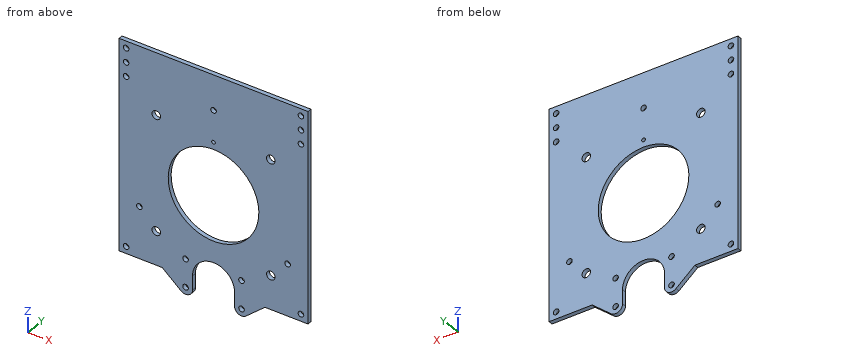
from build123d import *

# Parameters (mm, degrees)
SKETCH_1_R      = 2
SKETCH_1_R_2    = 3.05
SKETCH_1_R_3    = 1.3
SKETCH_1_R_4    = 32.4
EXTRUDE_1_DEPTH = 3


with BuildPart() as part:
    # ｽｹｯﾁ1 → ﾎﾞｽ - 押し出し1 (new body)
    with BuildSketch(Plane(origin=(0, 0, 0), x_dir=(1, 0, 0), z_dir=(0, 1, 0))):
        with BuildLine():
            Line((0, 150), (0, 0))
            Line((0, 0), (135, 0))
            Line((135, 0), (135, 150))
            Line((135, 150), (104.216771079, 150))
            Line((104.216771079, 150), (90.713938048, 161.330222216))
            ThreePointArc((90.713938048, 161.330222216), (85.386908691, 162.031538935), (82.5, 157.5))
            Line((82.5, 157.5), (82.5, 147.5))
            ThreePointArc((82.5, 147.5), (67.5, 132.5), (52.5, 147.5))
            Line((52.5, 147.5), (52.5, 150))
            Line((52.5, 150), (52.5, 157.5))
            ThreePointArc((52.5, 157.5), (49.613091309, 162.031538935), (44.286061952, 161.330222216))
            Line((44.286061952, 161.330222216), (30.783228921, 150))
            Line((30.783228921, 150), (0, 150))
        make_face()
        with Locations(Location((5, 5, 0), (0, 0, 270))):
            Circle(SKETCH_1_R, mode=Mode.SUBTRACT)
        with Locations(Location((5, 15, 0), (0, 0, 270))):
            Circle(SKETCH_1_R, mode=Mode.SUBTRACT)
        with Locations(Location((5, 25, 0), (0, 0, 270))):
            Circle(SKETCH_1_R, mode=Mode.SUBTRACT)
        with Locations(Location((26.558517369, 44.058517369, 0), (0, 0, 270))):
            Circle(SKETCH_1_R_2, mode=Mode.SUBTRACT)
        with Locations(Location((67.5, 25, 0), (0, 0, 270))):
            Circle(SKETCH_1_R, mode=Mode.SUBTRACT)
        with Locations(Location((130, 5, 0), (0, 0, 270))):
            Circle(SKETCH_1_R, mode=Mode.SUBTRACT)
        with Locations(Location((130, 15, 0), (0, 0, 270))):
            Circle(SKETCH_1_R, mode=Mode.SUBTRACT)
        with Locations(Location((130, 25, 0), (0, 0, 270))):
            Circle(SKETCH_1_R, mode=Mode.SUBTRACT)
        with Locations(Location((67.5, 47.5, 0), (0, 0, 270))):
            Circle(SKETCH_1_R_3, mode=Mode.SUBTRACT)
        with Locations(Location((108.441482631, 44.058517369, 0), (0, 0, 270))):
            Circle(SKETCH_1_R_2, mode=Mode.SUBTRACT)
        with Locations(Location((14.523144428, 113.168293767, 0), (0, 0, 270))):
            Circle(SKETCH_1_R, mode=Mode.SUBTRACT)
        with Locations(Location((67.5, 85, 0), (0, 0, 270))):
            Circle(SKETCH_1_R_4, mode=Mode.SUBTRACT)
        with Locations(Location((26.558517369, 125.941482631, 0), (0, 0, 270))):
            Circle(SKETCH_1_R_2, mode=Mode.SUBTRACT)
        with Locations(Location((5, 145, 0), (0, 0, 270))):
            Circle(SKETCH_1_R, mode=Mode.SUBTRACT)
        with Locations(Location((47.5, 137.5, 0), (0, 0, 270))):
            Circle(SKETCH_1_R, mode=Mode.SUBTRACT)
        with Locations(Location((47.5, 157.5, 0), (0, 0, 270))):
            Circle(SKETCH_1_R, mode=Mode.SUBTRACT)
        with Locations(Location((120.476855572, 113.168293767, 0), (0, 0, 270))):
            Circle(SKETCH_1_R, mode=Mode.SUBTRACT)
        with Locations(Location((87.5, 137.5, 0), (0, 0, 270))):
            Circle(SKETCH_1_R, mode=Mode.SUBTRACT)
        with Locations(Location((108.441482631, 125.941482631, 0), (0, 0, 270))):
            Circle(SKETCH_1_R_2, mode=Mode.SUBTRACT)
        with Locations(Location((130, 145, 0), (0, 0, 270))):
            Circle(SKETCH_1_R, mode=Mode.SUBTRACT)
        with Locations(Location((87.5, 157.5, 0), (0, 0, 270))):
            Circle(SKETCH_1_R, mode=Mode.SUBTRACT)
    extrude(amount=EXTRUDE_1_DEPTH)


solid = part.part
Work out the finished part from the listing and answer in its coordinate system (mm). Give positions to 0.01 mm unless a question says otherwise; leave off trailing zeros. Order: outer loops, then holes, each group sorted by start corner. A loop starts at its lowest first (then second) coordinate and runs counter-clockwise, first axis right, second up. Notation, with made-up numbers: (22.25, 13.25) -> (53.25, 13.25) arc R21 cw to (53.25, 45.25) -> close; hole circle Ø10 at (-30, 22.25). An arc over 180 degrees is marked (long way). Answer as a JSON object with one key per item and string values. Group by question number.
1. Consider line 1 along X through (y, z) = (2.15, -5); line 2 along X through (y, z) = (2.3, -125); line 3 along X through (y, z) = (2.4, -157.5). Determine where each line is inside the solid, lowest interval first. Write a range as [from, to].
2. Section B-B on x = 87.5 is taken. Determine the outline of the cut face in (y, z), plus the area to 3 significant figures.
3. Section D-D on z = -99.5 is taken. Determine the outline of the cut face in (x, y).
4. Section C-C on y = 0.75 is taken. Count the separate pieces of the cut face and the enclosed holes in it, plus the area to 3 significant figures.
5. Flat-ended cylindrical pins translate along their axes: pin 1 Ø3.5 at (x, z) = (26.56, -44.06) entering from +Y; pin 2 Ø0.9 at (y, z) = (1, -152.5) entering from +X; pin 3 Ø0.9 at (x, y) = (9.5, 1) entering from -Z. Find the tip coordinate at first contact, or state that the pin passes through.
6. Section A-A on z = -71 is taken. Determine the outline of the cut face in (x, y), plus the area to 3 significant figures.
Result sheet:
{
 "1": {"line 1": "x = [0, 3], [7, 128], [132, 135]", "line 2": "x = [0, 23.66], [29.46, 105.54], [111.34, 135]", "line 3": "x = [39.72, 45.5], [49.5, 52.5], [82.5, 85.5], [89.5, 95.28]"},
 "2": {"outline": "(0, -162.5) -> (3, -162.5) -> (3, -159.5) -> (0, -159.5) -> close; (0, -155.5) -> (3, -155.5) -> (3, -139.5) -> (0, -139.5) -> close; (0, -135.5) -> (3, -135.5) -> (3, -110.49) -> (0, -110.49) -> close; (0, -59.51) -> (3, -59.51) -> (3, 0) -> (0, 0) -> close", "area": "311 mm^2"},
 "3": {"outline": "(0, 0) -> (38.53, 0) -> (38.53, 3) -> (0, 3) -> close; (96.47, 0) -> (135, 0) -> (135, 3) -> (96.47, 3) -> close"},
 "4": {"separate pieces": "1", "enclosed holes": "21", "area": "16,600 mm^2"},
 "5": {"pin 1": "passes through", "pin 2": "stops at x = 101.77", "pin 3": "stops at z = -150"},
 "6": {"outline": "(0, 0) -> (38.28, 0) -> (38.28, 3) -> (0, 3) -> close; (96.72, 0) -> (135, 0) -> (135, 3) -> (96.72, 3) -> close", "area": "230 mm^2"}
}
